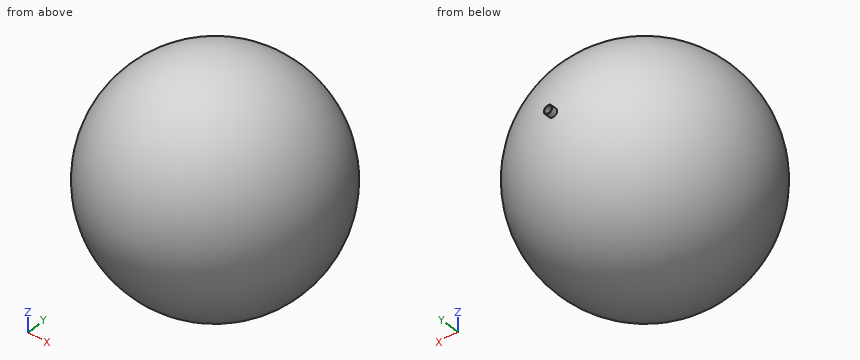
```python
from build123d import *

# Parameters (mm, degrees)
SKETCH76_R          = 30
BOSS_EXTRUDE1_DEPTH = 50
SKETCH78_R          = 25
CUT_EXTRUDE1_DEPTH  = 1378.239234241


with BuildPart() as part:
    # Sketch74 → Revolve4 (revolve)
    with BuildSketch(Plane.XY):
        with BuildLine():
            Line((0, 781.5925), (0, 771.5925))
            ThreePointArc((0, 771.5925), (771.5925, 0), (0, -771.5925))
            Line((0, -771.5925), (0, -781.5925))
            ThreePointArc((0, -781.5925), (781.5925, 0), (0, 781.5925))
        make_face()
    revolve(axis=Axis((0, 0, 0), (0, 1, 0)))

    # Sketch76 → Boss-Extrude1 (add)
    with BuildSketch(Plane(origin=(0, 771.5925, 0), x_dir=(1, 0, 0), z_dir=(0, 1, 0))):
        with Locations(Location((0, 0, 0), (0, 0, 90))):
            Circle(SKETCH76_R)
    extrude(amount=BOSS_EXTRUDE1_DEPTH)

    # Sketch78 → Cut-Extrude1 (cut, through all)
    with BuildSketch(Plane(origin=(0, 0, 0), x_dir=(1, 0, 0), z_dir=(0, 1, 0))):
        with Locations(Location((0, 0, 0), (0, 0, 90))):
            Circle(SKETCH78_R)
    extrude(amount=CUT_EXTRUDE1_DEPTH, mode=Mode.SUBTRACT)


solid = part.part
```
Verification items for the finished model (mm, model axes). Give positions to 0.01 mm unless a question says otherwise; leave off trailing zeros. Order: outer loops, then holes, each group sorted by start corner. A loop starts at its lowest first (then second) coordinate and runs counter-clockwise, first axis right, second up. Notation, with made-up numbers: (8, -2) -> (52, -2) arc R26 cw to (52, 12) -> close; hole circle Ø11 at (17, 49). An arc over 180 degrees is marked (long way). One line per item, written item: value.
(1) Sectioned sample at C-C on y = 41. Record the cut outline in (x, z).
Final values:
outline: circle Ø1561.03 at (0, 0); hole circle Ø1541 at (0, 0)
(2) Sectioned sample at A-A on x = 0. Record the cut outline in (y, z) (1 decimal), then the cut area to 3 significant figures.
Final values:
outline: (771.2, -25) arc R771.6 cw (long way) to (771.2, 25) -> (821.6, 25) -> (821.6, 30) -> (781, 30) arc R781.6 ccw (long way) to (781, -30) -> (821.6, -30) -> (821.6, -25) -> close
area: 48,700 mm^2
(3) Sectioned sample at B-B on z = 0. Record the cut outline in (x, y) (1 decimal).
Final values:
outline: (-30, 781) arc R781.6 ccw (long way) to (30, 781) -> (30, 821.6) -> (25, 821.6) -> (25, 771.2) arc R771.6 cw (long way) to (-25, 771.2) -> (-25, 821.6) -> (-30, 821.6) -> close
(4) Sectioned sample at D-D on z = 441. Record the cut outline in (x, y).
Final values:
outline: circle Ø1290.59 at (0, 0); hole circle Ø1266.29 at (0, 0)
(5) Gauge pin test, flat ends, axial feed: pin 1 (2 mm diameter, centred on y = -18.5, z = -414, fed in from -X); pin 2 (6 mm diameter, centred on x = 156, z = -30.5, fed in from +Y); pin 3 (5 mm diameter, centred on x = -310, z = -41, fed in from -Y). Record the tip position at first contact, or that the pin passes through.
Final values:
pin 1: x = -663.31
pin 2: y = 765.88
pin 3: y = -717.4
(6) Scan lines: line 1 along X through (y, z) = (789, 0); line 2 along Y through (x, z) = (37, -439.5); line 3 along X through (y, z) = (-420, 288.5). Record each from-to range of solid material in increasing order. Write a range as [from, to].
Final values:
line 1: [-30, -25], [25, 30]
line 2: [-645.26, -633.11], [633.11, 645.26]
line 3: [-592.67, -579.42], [579.42, 592.67]
